```python
from build123d import *

# Parameters (mm, degrees)
SALIENTE_EXTRUIR2_DEPTH   = 5
SALIENTE_EXTRUIR2_2_DEPTH = 5
SALIENTE_EXTRUIR2_3_DEPTH = 5
SALIENTE_EXTRUIR3_START   = -20
CROQUIS5_R                = 10
SALIENTE_EXTRUIR3_DEPTH   = 40
CROQUIS6_R                = 10
SALIENTE_EXTRUIR4_DEPTH   = 40
CROQUIS7_R                = 10
SALIENTE_EXTRUIR5_DEPTH   = 40


with BuildPart() as part:
    # Croquis4 → Saliente-Extruir2 (new body, symmetric)
    with BuildSketch(Plane(origin=(0, 0, 0), x_dir=(1, 0, 0), z_dir=(0, 1, 0))):
        Polygon((-303.846502665, -198.519870873), (-336.410161514, -217.320508076), (-331.410161514, -225.980762114), (331.410161514, -225.980762114), (336.410161514, -217.320508076), (303.846502665, -198.519870873), align=None)
    extrude(amount=SALIENTE_EXTRUIR2_DEPTH, both=True)



with BuildPart() as body_2:
    # Croquis4 → Saliente-Extruir2 2 (new body, symmetric)
    with BuildSketch(Plane(origin=(0, 0, 0), x_dir=(1, 0, 0), z_dir=(0, 1, 0))):
        Polygon((-20, 400), (-30, 400), (-361.410161514, -174.019237886), (-356.410161514, -182.679491924), (-323.846502665, -163.878854722), (-20, 362.398725595), align=None)
    extrude(amount=SALIENTE_EXTRUIR2_2_DEPTH, both=True)



with BuildPart() as body_3:
    # Croquis4 → Saliente-Extruir2 3 (new body, symmetric)
    with BuildSketch(Plane(origin=(0, 0, 0), x_dir=(1, 0, 0), z_dir=(0, 1, 0))):
        Polygon((30, 400), (20, 400), (20, 362.398725595), (323.846502665, -163.878854722), (356.410161514, -182.679491924), (361.410161514, -174.019237886), align=None)
    extrude(amount=SALIENTE_EXTRUIR2_3_DEPTH, both=True)


with BuildPart() as body_2_1:
    add(body_2.part)

    add(body_3.part)  # Saliente-Extruir3 merges body 3
    # Croquis5 → Saliente-Extruir3 (add)
    with BuildSketch(Plane(origin=(0, 0, 0), x_dir=(0, 0, -1), z_dir=(1, 0, 0)).offset(SALIENTE_EXTRUIR3_START)):
        with Locations((400, 0)):
            Circle(CROQUIS5_R)
    extrude(amount=SALIENTE_EXTRUIR3_DEPTH)


with BuildPart() as part_1:
    add(part.part)

    add(body_2_1.part)  # Saliente-Extruir4 merges body 2
    # Croquis6 → Saliente-Extruir4 (add)
    with BuildSketch(Plane(origin=(-10, 0, -17.320508076), x_dir=(0.866025404, 0, -0.5), z_dir=(0.5, 0, 0.866025404))):
        with Locations((-400, 0)):
            Circle(CROQUIS6_R)
    extrude(amount=SALIENTE_EXTRUIR4_DEPTH)

    # Croquis7 → Saliente-Extruir5 (add)
    with BuildSketch(Plane(origin=(10, 0, -17.320508076), x_dir=(0.866025404, 0, 0.5), z_dir=(-0.5, 0, 0.866025404))):
        with Locations((400, 0)):
            Circle(CROQUIS7_R)
    extrude(amount=SALIENTE_EXTRUIR5_DEPTH)


solid = part_1.part
```
Read the model definition and answer for the solid it produces. Units are mm, in the model's axes. A direction names the side the tool comes from. Give positions to 0.01 mm unless a question says otherwise; leave off trailing zeros. Order: outer loops, then holes, each group sorted by start corner. A loop starts at its lowest first (then second) coordinate and runs counter-clockwise, first axis right, second up. Notation, with made-up numbers: (-36, -6.5) -> (-3, -6.5) arc R28 ccw to (-3, 27.5) -> close; hole circle Ø11 at (82, 39.25). An arc over 180 degrees is marked (long way). One line per item, written item: value. Start each with the question number.
(1) A tool of negligible diameter and unlimited length cuts with its end or side. For faces 4 (the flat face through (169.8, 0.07, -102.94)), 5 (the flat face through (-193.385, 0.07, -117.009)), from which of +Z, -Z, +X, -X, +Y, -Y can it reach the whole face along a straight path? Write none if from no direction.
(2) Flat-ended cylindrical pins translate along their axes: P1, Ø13.5, axis at x = 157.5, z = 214, coming from the -Y side; P2, Ø8, axis at y = 2.5, z = -378.5, coming from the +X side; P3, Ø3, axis at y = 2, z = -378.5, coming from the -X side. Find the tip coordinate at first contact, or state that the pin passes through.
(3) The part is cut by section A-A (z = -279). Determine the outline of the cut face in (x, y), and give its area (3 significant figures).
(4) Straight lines are drawn through the part: L1, parallel to Z at x = -16.5, y = -0.25; L2, parallel to X at y = -2.25, z = -62.5; L3, parallel to Z at x = 185, y = -1. For each, find the intervals that lie inside material, in ascending order.
(5) For a pull along X with two mould halves and no side action, classify faces 1 (the flat face through (-192, -5, -88)), 2 (the cylindrical face through (354.81, 3, 204.53)), 3 (the flat face through (-358.899, 0.14, 184.116)) as released by +X, released by -X, zero draft, split by the parting line, or undercut.
(6) The part is cut by section B-B (x = 139.5). Determine the outline of the cut face in (y, z), and give its area (3 significant figures).
Taken from the geometry:
1. face 4: +Y, -Y
1. face 5: -Z, -X, +Y, -Y
2. P1: y = -5
2. P2: x = 44.72
2. P3: x = -43.28
3. outline: (-99.86, -5) -> (-68.15, -5) -> (-68.15, 5) -> (-99.86, 5) -> close; (68.15, -5) -> (99.86, -5) -> (99.86, 5) -> (68.15, 5) -> close
3. area: 634 mm^2
4. L1: -410 to -390, 198.52 to 225.98
4. L2: -224.86 to -193.15, 193.15 to 224.86
4. L3: -131.53 to -76.61, 198.52 to 225.98
5. face 1: zero draft
5. face 2: undercut
5. face 3: released by -X
6. outline: (-5, -210.34) -> (5, -210.34) -> (5, -155.42) -> (-5, -155.42) -> close; (-5, 198.52) -> (5, 198.52) -> (5, 225.98) -> (-5, 225.98) -> close
6. area: 824 mm^2
